Part model, mm, in its own coordinate system. Coordinates: 2 decimals unless noted, no trailing zeros. Loops run counter-clockwise (first coordinate to the right, second up) from the corner with the lowest first, then second, coordinate; pieces in that order, holes last. Notation, with made-up numbers: M 15.25,35.5 L 26.25,35.5 A17 cw 26.25,39.5 Z; hole C 76,88.5 d10. An arc over 180 degrees is marked long. Answer as a JSON object with one key per item and string values. Group by question number.
1. Drill centre lines: L1, parallel to Z at x = -32, y = -6; L2, parallel to X at y = -18, z = 35.5; L3, parallel to X at y = -19, z = 40. Where is each one in solid material? Low to high.
2. Saw through at C-C on z = 38.5. Write the cut outline in (x, y) (3 decimals).
3. Drop a flat-ended pin along its axis: pin 1 Ø12 at (x, y) = (-20.5, -14) entering from -Z. Give the stop position or say it passes through.
4. Saw through at A-A on y = -15.5. Write the cut outline in (x, z), then the cut area to 3 significant figures.
5. Saw through at B-B on x = -53.5. Write the cut outline in (y, z) (3 decimals).
from build123d import *

# Parameters (mm, degrees)
F1_DEPTH = 85.725
F2_R     = 7.62
F3_R     = 25.4
F4_R     = 25.4
F5_R     = 7.62


with BuildPart() as f1:
    # F0 (on Front) → F1 (new body)
    with BuildSketch(Plane.XZ):
        Polygon((-68.2625, 0), (0, 0), (68.2625, 0), (68.2625, 38.1), (38.1, 57.15), (0, 57.15), (-38.1, 57.15), (-68.2625, 38.1), align=None)
    extrude(amount=F1_DEPTH)

    # F2
    f2_edges = [f1.edges().sort_by_distance(p)[0] for p in [
        (-68.2625, -42.8625, 38.1),
    ]]
    fillet(f2_edges, radius=F2_R)

    # F3
    f3_edges = [f1.edges().sort_by_distance(p)[0] for p in [
        (-38.1, -42.8625, 57.15),
    ]]
    fillet(f3_edges, radius=F3_R)

    # F4
    f4_edges = [f1.edges().sort_by_distance(p)[0] for p in [
        (38.1, -42.8625, 57.15),
    ]]
    fillet(f4_edges, radius=F4_R)

    # F5
    f5_edges = [f1.edges().sort_by_distance(p)[0] for p in [
        (68.2625, -42.8625, 38.1),
    ]]
    fillet(f5_edges, radius=F5_R)


solid = f1.part
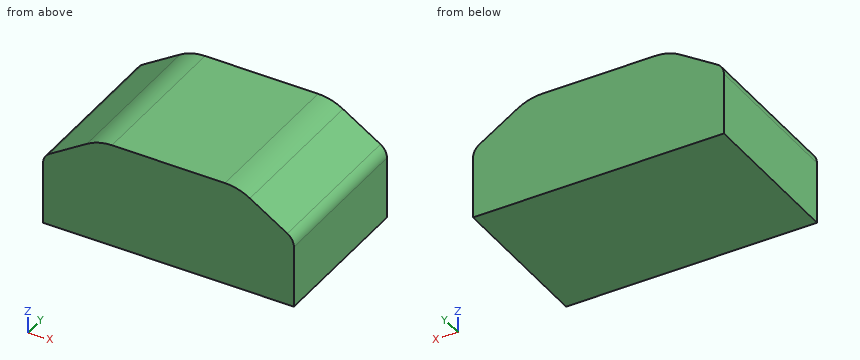
Outcome:
{
 "1": {"L1": "z = 0 to 57.12", "L2": "x = -68.09 to 68.09", "L3": "x = -65.21 to 65.21"},
 "2": {"outline": "M -66.717,-85.725 L 66.717,-85.725 L 66.717,0 L -66.717,0 Z"},
 "3": {"pin 1": "stops at z = 0"},
 "4": {"outline": "M -68.26,0 L 68.26,0 L 68.26,33.9 A7.62 ccw 64.71,40.34 L 44.31,53.23 A25.4 ccw 30.75,57.15 L -30.75,57.15 A25.4 ccw -44.31,53.23 L -64.71,40.34 A7.62 ccw -68.26,33.9 Z", "area": "7,210 mm²"},
 "5": {"outline": "M -85.725,0 L 0,0 L 0,47.424 L -85.725,47.424 Z"}
}
